```python
from build123d import *

# Parameters (mm, degrees)
SKETCH_1_W          = 40.5
SKETCH_1_H          = 19.9
EXTRUDE_1_DEPTH     = 28.25
SKETCH_2_W          = 54.15
SKETCH_2_H          = 19.9
EXTRUDE_2_DEPTH     = 2.4
SKETCH_3_W          = 40.5
SKETCH_3_H          = 19.9
EXTRUDE_3_DEPTH     = 6
SKETCH_4_R          = 9.95
SKETCH_4_W          = 19.601123737
SKETCH_4_H          = 17.8
EXTRUDE_4_DEPTH     = 1.8
SKETCH_5_R          = 6.55
EXTRUDE_5_DEPTH     = 1.8
SKETCH_6_R          = 1.6
EXTRUDE_6_DEPTH     = 4.5
SKETCH_7_R          = 2.25
CUT_EXTRUDE_1_DEPTH = 43.088960845
CHAMFER_1_SIZE      = 1


with BuildPart() as part:
    # 草图1 → 凸台-拉伸1 (new body)
    with BuildSketch(Plane(origin=(0, 0, 0), x_dir=(1, 0, 0), z_dir=(0, 1, 0))):
        Rectangle(SKETCH_1_W, SKETCH_1_H)
    extrude(amount=EXTRUDE_1_DEPTH)

    # 草图2 → 凸台-拉伸2 (add)
    with BuildSketch(Plane(origin=(0, 28.25, 0), x_dir=(1, 0, 0), z_dir=(0, 1, 0))):
        Rectangle(SKETCH_2_W, SKETCH_2_H)
    extrude(amount=EXTRUDE_2_DEPTH)

    # 草图3 → 凸台-拉伸3 (add)
    with BuildSketch(Plane(origin=(0, 30.65, 0), x_dir=(1, 0, 0), z_dir=(0, 1, 0))):
        Rectangle(SKETCH_3_W, SKETCH_3_H)
    extrude(amount=EXTRUDE_3_DEPTH)

    # 草图4 → 凸台-拉伸4 (add)
    with BuildSketch(Plane(origin=(0, 36.65, 0), x_dir=(1, 0, 0), z_dir=(0, 1, 0))):
        with Locations((10.3, 0)):
            Circle(SKETCH_4_R)
        with Locations((-3.949438132, 0)):
            Rectangle(SKETCH_4_W, SKETCH_4_H)
    extrude(amount=EXTRUDE_4_DEPTH)

    # 草图5 → 凸台-拉伸5 (add)
    with BuildSketch(Plane(origin=(0, 38.45, 0), x_dir=(1, 0, 0), z_dir=(0, 1, 0))):
        with Locations(Location((10.3, 0, 0), (0, 0, 270))):
            Circle(SKETCH_5_R)
    extrude(amount=EXTRUDE_5_DEPTH)

    # 草图6 → 凸台-拉伸6 (add)
    with BuildSketch(Plane(origin=(0, 40.25, 0), x_dir=(1, 0, 0), z_dir=(0, 1, 0))):
        with Locations(Location((10.3, 0, 0), (0, 0, 270))):
            Circle(SKETCH_6_R)
    extrude(amount=EXTRUDE_6_DEPTH)

    # 草图7 → 切除-拉伸1 (cut, through all)
    with BuildSketch(Plane(origin=(0, 30.65, 0), x_dir=(1, 0, 0), z_dir=(0, 1, 0))):
        with Locations(Location((24.45, -5.05, 0), (0, 0, 270))):
            Circle(SKETCH_7_R)
        with Locations(Location((24.45, 5.05, 0), (0, 0, 270))):
            Circle(SKETCH_7_R)
        with Locations(Location((-24.45, 5.05, 0), (0, 0, 270))):
            Circle(SKETCH_7_R)
        with Locations(Location((-24.45, -5.05, 0), (0, 0, 270))):
            Circle(SKETCH_7_R)
    extrude(amount=-CUT_EXTRUDE_1_DEPTH, mode=Mode.SUBTRACT)

    # 倒角1
    chamfer_1_edges = [part.edges().sort_by_distance(p)[0] for p in [
        (0, 0, 9.95),
        (-20.25, 0, 0),
        (0, 0, -9.95),
        (20.25, 0, 0),
    ]]
    chamfer(chamfer_1_edges, length=CHAMFER_1_SIZE)


solid = part.part
```
Model file for the job. Use its own axes, mm. A direction names the side the tool comes from. Coordinates: 2 decimals unless noted, no trailing zeros. Order: outer loops, then holes, each group sorted by start corner. A loop starts at its lowest first (then second) coordinate and runs counter-clockwise, first axis right, second up. Notation, with made-up numbers: (28.5, 75) -> (57.5, 75) arc R11 ccw to (57.5, 90) -> close; hole circle Ø5 at (-22, -31.5). An arc over 180 degrees is marked (long way). Return JSON: item names as keys, results as strings.
Item 1: Mould opens along X. For faces 1 (the face through (22.254, 29.467, 4.562)), 2 (the face through (-4, 38, -8.9)), 3 (the face through (-27.075, 29, 0)), 4 (the face through (-26.646, 29.467, 4.562)) say: pulls with the +X half, pulls with the -X half, needs draft (parallel to the pull), parting line crosses it, or undercut.
Model answer:
{"face 1": "undercut", "face 2": "needs draft", "face 3": "pulls with the -X half", "face 4": "undercut"}
Item 2: Slice it at D-D (y = 10). Write the cut outline in (x, z).
Model answer:
{"outline": "(-20.25, -9.95) -> (20.25, -9.95) -> (20.25, 9.95) -> (-20.25, 9.95) -> close"}
Item 3: Slice it at A-A (x = 24.45). Write the cut outline in (y, z), then the cut area to 3 significant figures.
Model answer:
{"outline": "(28.25, -9.95) -> (30.65, -9.95) -> (30.65, -7.3) -> (28.25, -7.3) -> close; (28.25, -2.8) -> (30.65, -2.8) -> (30.65, 2.8) -> (28.25, 2.8) -> close; (28.25, 7.3) -> (30.65, 7.3) -> (30.65, 9.95) -> (28.25, 9.95) -> close", "area": "26.2 mm²"}
Item 4: Slice it at C-C (x = 1). Write the cut outline in (y, z).
Model answer:
{"outline": "(0, -8.95) -> (1, -9.95) -> (36.65, -9.95) -> (36.65, -8.9) -> (38.45, -8.9) -> (38.45, 8.9) -> (36.65, 8.9) -> (36.65, 9.95) -> (1, 9.95) -> (0, 8.95) -> close"}
Item 5: Slice it at B-B (z = 4). Count the separate pieces of the cut face and the enclosed holes in it, then the cut area to 3 significant figures.
Model answer:
{"separate pieces": "3", "enclosed holes": "0", "area": "1,580 mm²"}
Item 6: Wall check: line 1 along X through (y, z) = (29.5, -5) (3 decimals); line 2 along Y through (x, z) = (-15.5, 0); line 3 along Y through (x, z) = (-6, 2.5). Give the ranges that are in metal, low to high. Write a range as from..to.
Model answer:
{"line 1": "x = -27.075..-26.699, -22.201..22.201, 26.699..27.075", "line 2": "y = 0..36.65", "line 3": "y = 0..38.45"}
Item 7: Pin check, flat tips, straight feed: P1, Ø6, axis at x = -24.45, z = -5.05, coming from the +Y side; P2, Ø0.9, axis at x = -0.5, y = 37.5, coming from the -Z side; P3, Ø11, axis at x = 15, z = -7.5, coming from the +Y side. Stop position of each tip, or through.
Model answer:
{"P1": "stops at y = 30.65", "P2": "stops at z = -8.9", "P3": "stops at y = 40.25"}
Item 8: 3-axis set-ups, long thin cutter, end or side, ignore diameter. For faces 5 (the face through (-24, 28.25, 0)), 6 (the face through (18, 36.65, -8)), 7 (the face through (-13.75, 38, 0)), 8 (the face through (20.25, 34, 0)), 9 (the face through (8.9, 40.25, 1.4)): which of +Z, -Z, +X, -X, +Y, -Y reach the whole face in a straight line?
Model answer:
{"face 5": "+Z, -Z, -X, -Y", "face 6": "-Z, +X, +Y", "face 7": "+Z, -Z, -X, +Y", "face 8": "+Z, -Z, +X, +Y", "face 9": "+Y"}
